Read the model definition and answer for the solid it produces. Units are mm, in the model's axes. A direction names the side the tool comes from. Coordinates: 2 decimals unless noted, no trailing zeros. Write each loop counter-clockwise with the first axis right and the second up, starting at its lowest first coordinate (ties: lowest second). Pieces come first, ordered by that corner, then holes. Notation, with made-up numbers: (-24.75, 60.25) -> (29.25, 60.25) arc R11 cw to (29.25, 70.25) -> close; hole circle Ø1 at (-17.5, 56). An arc over 180 degrees is marked (long way). Answer as a JSON object with one key per item and string values. Group by question number.
(1) Find section D-D (x = 0). Give the vertices of the cut face in (y, z), then the cut area to 3 significant figures.
(2) Find section B-B (y = 0). Give the vertices of the cut face in (x, z) (3 decimals), then the cut area to 3 significant figures.
(3) Which of the six approach directions +Z, -Z, +X, -X, +Y, -Y give full straight-line access (tool end or side, diameter ignored) to faces 5 (the face through (3.875, 0, 6)), 6 (the face through (23, 4, 2)), 7 (the face through (22.346, 0, 2))?
(4) Straight lines are drawn through the part: L1, parallel to Y at x = 0, z = 1.4; L2, parallel to X at y = -6, z = 6 (3 decimals); L3, parallel to X at y = -17.5, z = 4.25 (3 decimals). For each, find the intervals that lie inside material, in ascending order.
(5) Flat-ended cylindrical pins translate along their axes: P1, Ø1.5, axis at y = 14, z = 5, coming from the -X side; P2, Ø3, axis at x = 22, z = 2, coming from the +Y side; P3, Ø1.9, axis at x = 21, z = 1.5, coming from the -Y side; P4, Ø3.5, axis at x = 0, y = 0, coming from the +Z side. Find the tip coordinate at first contact, or state that the pin passes through.
(6) For a pull along Y with two mould halves and no side action, classify faces 1 (the face through (23, 0, 4)), 2 (the face through (21, 1.5, 2)), 3 (the face through (22, -4, 2)), 4 (the face through (21, -1.5, 2)) as +Y half, -Y half, draft (parallel to the pull), parting line (faces both ways), or undercut.
(7) Find section A-A (x = 21.5). Give the vertices of the cut face in (y, z), then the cut area to 3 significant figures.
(8) Find section C-C (z = 6.75). Give the vertices of the cut face in (x, y) (3 decimals).
from build123d import *

# Parameters (mm, degrees)
F0_R     = 20
F1_DEPTH = 7.75
F2_W     = 7.75
F2_H     = 40
F3_DEPTH = 4.5
F5_DEPTH = 4
F6_R     = 2.8
F7_DEPTH = 3.251


with BuildPart() as f1:
    # F0 (on Top) → F1 (new body)
    with BuildSketch(Plane.XY):
        Circle(F0_R)
    extrude(amount=F1_DEPTH)

    # F2 (on face) → F3 (cut)
    with BuildSketch(Plane.XY.offset(7.75)):
        Rectangle(F2_W, F2_H)
    extrude(amount=-F3_DEPTH, mode=Mode.SUBTRACT)

    # F4 (on Top) → F5 (join)
    with BuildSketch(Plane.XY):
        Polygon((22.345918, -1.5), (18.466113, -1.5), (19.595918, -4), (24.845918, -4), (24.845918, 4), (20.595918, 4), (20.595918, 1.5), (22.345918, 1.5), align=None)
    extrude(amount=F5_DEPTH)

    # F6 (on face) → F7 (cut, through all)
    with BuildSketch(Plane.XY.offset(3.25)):
        Circle(F6_R)
    extrude(amount=-F7_DEPTH, mode=Mode.SUBTRACT)


solid = f1.part
Results below:
{
 "1": {"outline": "(-20, 0) -> (-2.8, 0) -> (-2.8, 3.25) -> (-20, 3.25) -> close; (2.8, 0) -> (20, 0) -> (20, 3.25) -> (2.8, 3.25) -> close", "area": "112 mm2"},
 "2": {"outline": "(-20, 0) -> (-2.8, 0) -> (-2.8, 3.25) -> (-3.875, 3.25) -> (-3.875, 7.75) -> (-20, 7.75) -> close; (2.8, 0) -> (20, 0) -> (20, 7.75) -> (3.875, 7.75) -> (3.875, 3.25) -> (2.8, 3.25) -> close; (22.346, 0) -> (24.846, 0) -> (24.846, 4) -> (22.346, 4) -> close", "area": "267 mm2"},
 "3": {"face 5": "+Z, +Y, -Y", "face 6": "+Z, -Z, +X, +Y", "face 7": "+Z, -Z"},
 "4": {"L1": "y = -20 to -2.8, 2.8 to 20", "L2": "x = -19.079 to -3.875, 3.875 to 19.079", "L3": "x = -9.682 to -3.875, 3.875 to 9.682"},
 "5": {"P1": "stops at x = -14.98", "P2": "stops at y = 4", "P3": "stops at y = -4", "P4": "passes through"},
 "6": {"face 1": "draft", "face 2": "undercut", "face 3": "-Y half", "face 4": "undercut"},
 "7": {"outline": "(-4, 0) -> (-1.5, 0) -> (-1.5, 4) -> (-4, 4) -> close; (1.5, 0) -> (4, 0) -> (4, 4) -> (1.5, 4) -> close", "area": "20.0 mm2"},
 "8": {"outline": "(-3.875, -19.621) -> (-3.875, 19.621) arc R20 ccw to start; (3.875, -19.621) arc R20 ccw to (3.875, 19.621) -> close"}
}
